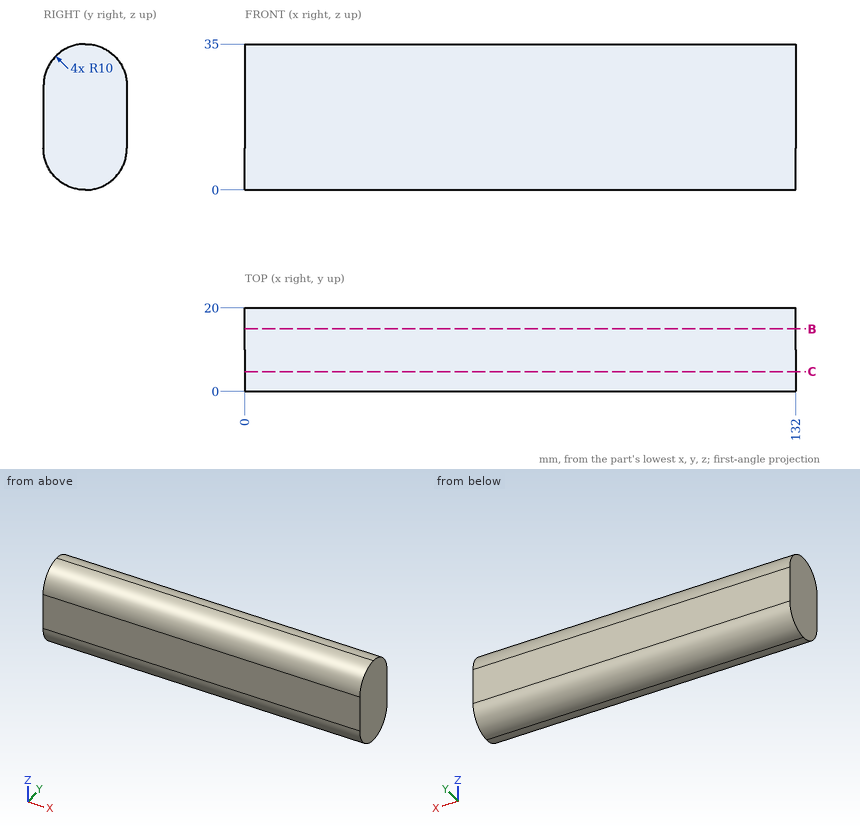
Part print with two shaded views. Sizes in mm from the minimum x, y, z corner. Coordinates: 2 decimals unless noted, no trailing zeros. Order: outer loops, then holes, each group sorted by start corner. A loop starts at its lowest first (then second) coordinate and runs counter-clockwise, first axis right, second up. Notation, with made-up numbers: M 35,-26.75 L 89,-26.75 A28 cw 89,9.25 Z; hole C 56,44 d1. An arc over 180 degrees is marked long. One line per question, with ' | ' between items. Start each with the question number.
1. Flat gauge pin, fed straight in: P1, Ø3, axis at x = 47, y = 16.5, coming from the +Z side. Where does the tip first touch, or does it go through?
2. Cut at C-C (y = 4.75). Write the cut outline in (x, z).
3. Cut at B-B (y = 15). Write the cut outline in (x, z), plus the area to 3 significant figures.
4. Wall check: line 1 along Z through (x, y) = (28.5, 14.75); line 2 along Y through (x, z) = (111, 8.5); line 3 along Z through (x, y) = (111.5, 16.5). Give the ranges that are in metal, low to high. Write a range as [from, to].
The answers:
1) P1: stops at z = 33.66
2) outline: M 0,1.49 L 132,1.49 L 132,33.51 L 0,33.51 Z
3) outline: M 0,1.34 L 132,1.34 L 132,33.66 L 0,33.66 Z | area: 4,270 mm2
4) line 1: z = [1.2, 33.8] | line 2: y = [0.11, 19.89] | line 3: z = [2.4, 32.6]
